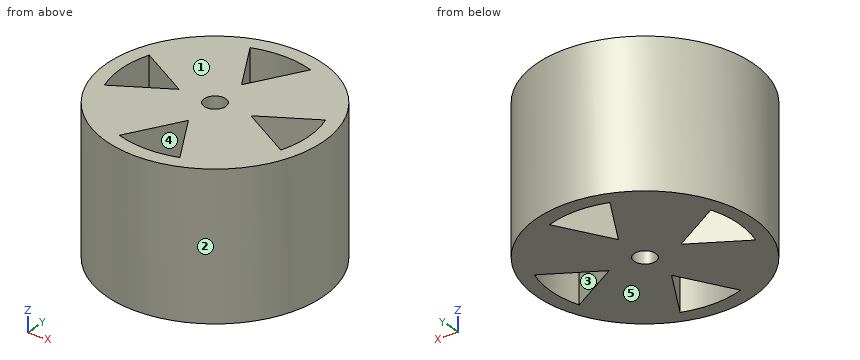
from build123d import *

# Parameters (mm, degrees)
SKETCH1_R           = 7.5
SKETCH1_R_2         = 0.75
BOSS_EXTRUDE1_DEPTH = 10
CUT_EXTRUDE1_DEPTH  = 11


with BuildPart() as part:
    # Sketch1 → Boss-Extrude1 (new body)
    with BuildSketch(Plane.XY):
        Circle(SKETCH1_R)
        Circle(SKETCH1_R_2, mode=Mode.SUBTRACT)
    extrude(amount=BOSS_EXTRUDE1_DEPTH)

    # Sketch2 → Cut-Extrude1 (cut, through all)
    with BuildSketch(Plane.XY.offset(10)):
        with BuildLine():
            Line((2.106805951, -6.149094948), (0, -2.5))
            Line((0, -2.5), (-2.106805951, -6.149094948))
            ThreePointArc((-2.106805951, -6.149094948), (0, -6.5), (2.106805951, -6.149094948))
        make_face()
        with BuildLine():
            Line((-6.149094948, -2.106805951), (-2.5, 0))
            Line((-2.5, 0), (-6.149094948, 2.106805951))
            ThreePointArc((-6.149094948, 2.106805951), (-6.5, 0), (-6.149094948, -2.106805951))
        make_face()
        with BuildLine():
            Line((6.149094948, 2.106805951), (2.5, 0))
            Line((2.5, 0), (6.149094948, -2.106805951))
            ThreePointArc((6.149094948, -2.106805951), (6.5, 0), (6.149094948, 2.106805951))
        make_face()
        with BuildLine():
            Line((-2.106805951, 6.149094948), (0, 2.5))
            Line((0, 2.5), (2.106805951, 6.149094948))
            ThreePointArc((2.106805951, 6.149094948), (0, 6.5), (-2.106805951, 6.149094948))
        make_face()
    extrude(amount=-CUT_EXTRUDE1_DEPTH, mode=Mode.SUBTRACT)


solid = part.part
Work out the finished part from the listing and answer in its coordinate system (mm). Face numbers are marked on the shaded views. A direction names the side the tool comes from. Round coordinates to 2 decimals unless told otherwise and drop trailing zeros. Write each loop counter-clockwise with the first axis right and the second up, starting at its lowest first coordinate (ties: lowest second). Pieces come first, ordered by that corner, then holes. Notation, with made-up numbers: (35.25, 89.25) - (49.25, 89.25) arc R14 cw to (49.25, 114.25) - close; hole circle Ø6 at (62.25, -16). An arc over 180 degrees is marked (long way). Answer in a Markdown table with one row per item. Add a question column.
1. The mould has two halves that part along Y. Classify the marked faces 1, 2 and 3: +Y half, -Y half, draft (parallel to the pull), parting line (faces both ways), or undercut.
2. A cutting plane is placed at D-D, the plane y = 4. Determine the outline of the cut face in (x, z), and give its area (3 significant figures).
3. A cutting plane is placed at B-B, the plane y = 0.5. Determine the outline of the cut face in (x, z).
4. A cutting plane is placed at C-C, the plane x = 4.5. Determine the outline of the cut face in (y, z).
5. Find the intervals of material crossed by line 1 along Y through (x, z) = (-1, 7.5); line 2 along Y through (x, z) = (-1.5, 8); line 3 along Y through (x, z) = (5.25, 1), in increasing order. Write a range as from..to.
6. For the marked faces 4 and 5, determine the directions among +Z, -Z, +X, -X, +Y, -Y from which every point of the face is accessible in a straight line to the end or side of a thin tool.
7. A cutting plane is placed at A-A, the plane z = 3.5. Determine the outline of the cut face in (x, y), and give its area (3 significant figures).
Worked out:
| question | item | result |
|---|---|---|
| 1 | face 1 | draft |
| 1 | face 2 | parting line |
| 1 | face 3 | undercut |
| 2 | outline | (-6.34, 0) - (-0.87, 0) - (-0.87, 10) - (-6.34, 10) - close; (0.87, 0) - (6.34, 0) - (6.34, 10) - (0.87, 10) - close |
| 2 | area | 110 mm^2 |
| 3 | outline | (-7.48, 0) - (-6.48, 0) - (-6.48, 10) - (-7.48, 10) - close; (-3.37, 0) - (-0.56, 0) - (-0.56, 10) - (-3.37, 10) - close; (0.56, 0) - (3.37, 0) - (3.37, 10) - (0.56, 10) - close; (6.48, 0) - (7.48, 0) - (7.48, 10) - (6.48, 10) - close |
| 4 | outline | (-6, 0) - (-1.15, 0) - (-1.15, 10) - (-6, 10) - close; (1.15, 0) - (6, 0) - (6, 10) - (1.15, 10) - close |
| 5 | line 1 | -7.43..-6.42, -4.23..4.23, 6.42..7.43 |
| 5 | line 2 | -7.35..-6.32, -5.1..5.1, 6.32..7.35 |
| 5 | line 3 | -5.36..-1.59, 1.59..5.36 |
| 6 | face 4 | +Z, -Z |
| 6 | face 5 | -Z, +X, -X, +Y, -Y |
| 7 | outline | circle Ø15 at (0, 0); hole (-6.15, -2.11) - (-2.5, 0) - (-6.15, 2.11) arc R6.5 ccw to start; hole (-2.11, -6.15) arc R6.5 ccw to (2.11, -6.15) - (0, -2.5) - close; hole (-2.11, 6.15) - (0, 2.5) - (2.11, 6.15) arc R6.5 ccw to start; hole circle Ø1.5 at (0, 0); hole (2.5, 0) - (6.15, -2.11) arc R6.5 ccw to (6.15, 2.11) - close |
| 7 | area | 140 mm^2 |
